```python
from build123d import *

# Parameters (mm, degrees)
SKETCH1_R           = 2.5
SKETCH1_R_2         = 1.5
SKETCH1_R_3         = 4.5
BOSS_EXTRUDE1_DEPTH = 3


with BuildPart() as part:
    # Sketch1 → Boss-Extrude1 (new body)
    with BuildSketch(Plane(origin=(0, 0, 0), x_dir=(1, 0, 0), z_dir=(0, 1, 0))):
        with BuildLine():
            Line((-188, -80), (188, -80))
            ThreePointArc((188, -80), (196.485281374, -76.485281374), (200, -68))
            Line((200, -68), (200, 68))
            ThreePointArc((200, 68), (196.485281374, 76.485281374), (188, 80))
            Line((188, 80), (-188, 80))
            ThreePointArc((-188, 80), (-196.485281374, 76.485281374), (-200, 68))
            Line((-200, 68), (-200, -68))
            ThreePointArc((-200, -68), (-196.485281374, -76.485281374), (-188, -80))
        make_face()
        with Locations(Location((-188, 68, 0), (0, 0, 270))):
            Circle(SKETCH1_R, mode=Mode.SUBTRACT)
        with Locations(Location((0, 68, 0), (0, 0, 270))):
            Circle(SKETCH1_R, mode=Mode.SUBTRACT)
        with Locations(Location((188, 68, 0), (0, 0, 270))):
            Circle(SKETCH1_R, mode=Mode.SUBTRACT)
        with Locations(Location((188, -68, 0), (0, 0, 270))):
            Circle(SKETCH1_R, mode=Mode.SUBTRACT)
        with Locations(Location((0, -68, 0), (0, 0, 270))):
            Circle(SKETCH1_R, mode=Mode.SUBTRACT)
        with Locations(Location((-188, -68, 0), (0, 0, 270))):
            Circle(SKETCH1_R, mode=Mode.SUBTRACT)
        with Locations(Location((-21.5, 52.5, 0), (0, 0, 270))):
            Circle(SKETCH1_R_2, mode=Mode.SUBTRACT)
        with Locations(Location((-21.5, -2.5, 0), (0, 0, 270))):
            Circle(SKETCH1_R_2, mode=Mode.SUBTRACT)
        with Locations(Location((69, 4, 0), (0, 0, 270))):
            Circle(SKETCH1_R_2, mode=Mode.SUBTRACT)
        with Locations(Location((88, 4, 0), (0, 0, 270))):
            Circle(SKETCH1_R_2, mode=Mode.SUBTRACT)
        with Locations(Location((69, -68, 0), (0, 0, 270))):
            Circle(SKETCH1_R_2, mode=Mode.SUBTRACT)
        with Locations(Location((88, -68, 0), (0, 0, 270))):
            Circle(SKETCH1_R_2, mode=Mode.SUBTRACT)
        with Locations(Location((-133, 32, 0), (0, 0, 270))):
            Circle(SKETCH1_R_3, mode=Mode.SUBTRACT)
        with Locations(Location((-164, 64, 0), (0, 0, 270))):
            Circle(SKETCH1_R, mode=Mode.SUBTRACT)
        with Locations(Location((-102, 64, 0), (0, 0, 270))):
            Circle(SKETCH1_R, mode=Mode.SUBTRACT)
        with Locations(Location((-102, 0, 0), (0, 0, 270))):
            Circle(SKETCH1_R, mode=Mode.SUBTRACT)
        with Locations(Location((-164, 0, 0), (0, 0, 270))):
            Circle(SKETCH1_R, mode=Mode.SUBTRACT)
        with BuildLine():
            Line((-2.5, -59), (159.5, -59))
            ThreePointArc((159.5, -59), (161.621320344, -58.121320344), (162.5, -56))
            Line((162.5, -56), (162.5, -15))
            ThreePointArc((162.5, -15), (161.621320344, -12.878679656), (159.5, -12))
            Line((159.5, -12), (-2.5, -12))
            ThreePointArc((-2.5, -12), (-4.621320344, -12.878679656), (-5.5, -15))
            Line((-5.5, -15), (-5.5, -56))
            ThreePointArc((-5.5, -56), (-4.621320344, -58.121320344), (-2.5, -59))
        make_face(mode=Mode.SUBTRACT)
    extrude(amount=BOSS_EXTRUDE1_DEPTH)


solid = part.part
```
Check sheet for the modelled part. Datum: model origin and axes. Units: mm. Round coordinates to 2 decimals unless told otherwise and drop trailing zeros. Order: outer loops, then holes, each group sorted by start corner. A loop starts at its lowest first (then second) coordinate and runs counter-clockwise, first axis right, second up. Notation, with made-up numbers: (50.25, 45.5) - (105.25, 45.5) arc R15 ccw to (105.25, 49.5) - close; hole circle Ø4 at (26.25, 80.5). An arc over 180 degrees is marked (long way). Write item = value, one per line.
Q1. Draft check along X on faces 1 (the face through (-196.58, 1.48, 76.39)), 2 (the face through (196.58, 1.48, -76.39)), 3 (the face through (-137.39, 1.48, -32.98)), 4 (the face through (-3, 0, -1)). Enter one of: pulls with the +X half, pulls with the -X half, needs draft (parallel to the pull), parting line crosses it, or undercut.
Computed:
face_1 = pulls with the -X half
face_2 = pulls with the +X half
face_3 = undercut
face_4 = needs draft
Q2. Section check A-A (x = 153). Record the boundary of the cut face in (y, z).
Computed:
outline = (0, -80) - (3, -80) - (3, 12) - (0, 12) - close; (0, 59) - (3, 59) - (3, 80) - (0, 80) - close
Q3. Section check C-C (z = 30.5). Record the boundary of the cut face in (x, y), and give its area (3 significant figures).
Computed:
outline = (-200, 0) - (-5.5, 0) - (-5.5, 3) - (-200, 3) - close; (162.5, 0) - (200, 0) - (200, 3) - (162.5, 3) - close
area = 696 mm^2
Q4. Thickness scan on line 1 along X through (y, z) = (1.3, 68); line 2 along Z through (x, y) = (-188, 1.65); line 3 along Z through (x, y) = (88, 1.3). Record the ranges inside material, lowest first.
Computed:
line_1 = -200 to -190.5, -185.5 to -2.5, 2.5 to 67.5, 70.5 to 86.5, 89.5 to 185.5, 190.5 to 200
line_2 = -80 to -70.5, -65.5 to 65.5, 70.5 to 80
line_3 = -80 to -5.5, -2.5 to 12, 59 to 66.5, 69.5 to 80
Q5. Section check B-B (y = 0.5). State how many separate pieces and enclosed holes the cut face has, and give its area (3 significant figures).
Computed:
separate_pieces = 1
enclosed_holes = 18
area = 55,700 mm^2
